```python
from build123d import *

# Parameters (mm, degrees)
SKETCH1_R           = 1.3
SKETCH1_R_2         = 0.3
BOSS_EXTRUDE1_DEPTH = 1
SKETCH1_3_R         = 0.765
BOSS_EXTRUDE2_DEPTH = 0.7
BOSS_EXTRUDE3_DEPTH = 0.6
BOSS_EXTRUDE4_DEPTH = 0.6
BOSS_EXTRUDE5_DEPTH = 0.4
SKETCH5_R           = 0.3
BOSS_EXTRUDE6_DEPTH = 0.4


with BuildPart() as part:
    # Sketch1 → Boss-Extrude1 (new body, symmetric)
    with BuildSketch(Plane.XY):
        Circle(SKETCH1_R)
        Circle(SKETCH1_R_2, mode=Mode.SUBTRACT)
    extrude(amount=BOSS_EXTRUDE1_DEPTH, both=True)



with BuildPart() as body_2:
    # Sketch1_3 → Boss-Extrude2 (new body, symmetric)
    with BuildSketch(Plane.XY):
        with Locations((3.98, -0.68)):
            Circle(SKETCH1_3_R)
    extrude(amount=BOSS_EXTRUDE2_DEPTH, both=True)


with BuildPart() as part_1:
    add(part.part)

    add(body_2.part)  # Boss-Extrude3 merges body 2
    # Sketch1_4 → Boss-Extrude3 (add, symmetric)
    with BuildSketch(Plane.XY):
        with BuildLine():
            ThreePointArc((3.663511304, -1.376462422), (3.215, -0.68), (3.663511304, 0.016462422))
            Line((3.663511304, 0.016462422), (2.68078674, 0.677070497))
            Line((2.68078674, 0.677070497), (0.521604487, 1.190768138))
            ThreePointArc((0.521604487, 1.190768138), (1.088137361, 0.711306603), (1.3, 0))
            ThreePointArc((1.3, 0), (1.133486255, -0.636560217), (0.676601677, -1.110049626))
            add(Edge.make_bspline(
                [(3.663511304, -1.376462422), (2.756337447, -0.967349054), (1.621818, -0.614489974), (0.676601677, -1.110049626)],
                knots=[0, 0, 0, 0, 1, 1, 1, 1], degree=3))
        make_face()
    extrude(amount=BOSS_EXTRUDE3_DEPTH, both=True)

    # Sketch1_5 → Boss-Extrude4 (add, symmetric)
    with BuildSketch(Plane.XY):
        with BuildLine():
            ThreePointArc((-1.295745132, -0.105093068), (-1.071749439, 0.735767042), (-0.36754671, 1.24696007))
            Line((-0.36754671, 1.24696007), (-2.029761859, 2.388087912))
            Line((-2.029761859, 2.388087912), (-3.468005165, 2.793231136))
            Line((-3.468005165, 2.793231136), (-3.852867925, 2.232623737))
            Line((-3.852867925, 2.232623737), (-2.957960282, 1.036034774))
            Line((-2.957960282, 1.036034774), (-1.295745132, -0.105093068))
        make_face()
    extrude(amount=BOSS_EXTRUDE4_DEPTH, both=True)



with BuildPart() as body_2_2:
    # Sketch2 → Revolve1 (revolve)
    with BuildSketch(Plane.XY):
        with BuildLine():
            Line((-3.852867925, 2.232623737), (-3.445366179, 2.826208042))
            Line((-3.445366179, 2.826208042), (-3.775135237, 3.052597901))
            Line((-3.775135237, 3.052597901), (-4.815155649, 1.537660116))
            ThreePointArc((-4.815155649, 1.537660116), (-4.383926247, 1.56515911), (-4.30804714, 1.990549933))
            Line((-4.30804714, 1.990549933), (-3.852867925, 2.232623737))
        make_face()
    revolve(axis=Axis((-3.775135237, 3.052597901, 0), (-0.565974648, -0.824422645, 0)))


with BuildPart() as part_2:
    add(part_1.part)

    add(body_2_2.part)  # Revolve2 merges body 2 2
    # Sketch3 → Revolve2 (revolve)
    with BuildSketch(Plane.XY):
        Polygon((-3.6732598, 3.200993977), (-4.28451242, 2.31061752), (-5.034737027, 2.82565445), (-4.423484407, 3.716030906), align=None)
    revolve(axis=Axis((-3.6732598, 3.200993977, 0), (-0.565974648, -0.824422645, 0)))

    # Sketch4 → Boss-Extrude5 (add)
    with BuildSketch(Plane(origin=(0.316945803, 0.461676681, 0), x_dir=(0.824422645, -0.565974648, 0), z_dir=(0.565974648, 0.824422645, 0))):
        Polygon((-4.84, 0.75055535), (-5.49, 0.375277675), (-5.49, -0.375277675), (-4.84, -0.75055535), (-4.19, -0.375277675), (-4.19, 0.375277675), align=None)
    extrude(amount=BOSS_EXTRUDE5_DEPTH)

    # Sketch5 → Boss-Extrude6 (add)
    with BuildSketch(Plane(origin=(0.543335662, 0.791445739, 0), x_dir=(0.824422645, -0.565974648, 0), z_dir=(0.565974648, 0.824422645, 0))):
        with Locations((-4.84, 0)):
            Circle(SKETCH5_R)
    extrude(amount=BOSS_EXTRUDE6_DEPTH)


solid = part_2.part
```
Geometry: final body of the model. Coordinates: model frame, mm. A direction names the side the tool comes from. Give positions to 0.01 mm unless a question says otherwise; leave off trailing zeros. Loops run counter-clockwise (first coordinate to the right, second up) from the corner with the lowest first, then second, coordinate; pieces in that order, holes last. Notation, with made-up numbers: (24, -14.75) -> (83, -14.75) arc R11 ccw to (83, 2.25) -> close; hole circle Ø3 at (72, -39.5). An arc over 180 degrees is marked (long way). Return JSON: item names as keys, results as strings.
Item 1: Section D-D, the plane y = -0.45. Output: boundary loops of the cut face in (x, z), plus the area to 3 significant figures.
Filled in:
{"outline": "(-1.22, -1) -> (1.22, -1) -> (1.22, -0.6) -> (3.25, -0.6) -> (3.25, -0.7) -> (4.71, -0.7) -> (4.71, 0.7) -> (3.25, 0.7) -> (3.25, 0.6) -> (1.22, 0.6) -> (1.22, 1) -> (-1.22, 1) -> close", "area": "9.36 mm^2"}
Item 2: Access query for faces 1 (the flat face through (4, -1, -0.7)), 2 (the flat face through (4, -1, 0.7)), 3 (the cylindrical face through (-0.28, -1.27, 0.01)). Directions: +Z, -Z, +X, -X, +Y, -Y. A direction counts if a zero-diameter tool reaches every point of the face in a straight line with its end or side. Return the directions, or none.
Filled in:
{"face 1": "-Z, +X, +Y, -Y", "face 2": "+Z, +X, +Y, -Y", "face 3": "none"}
Item 3: Section A-A, the plane x = 0. Output: boundary loops of the cut face in (y, z).
Filled in:
{"outline": "(-1.3, -1) -> (-0.3, -1) -> (-0.3, 1) -> (-1.3, 1) -> close; (0.3, -1) -> (1.3, -1) -> (1.3, 1) -> (0.3, 1) -> close"}
Item 4: Pin query (flat end, axial travel): P1, Ø0.5, axis at x = 4, y = -1, coming from the +Z side; P2, Ø2.5, axis at x = -2.5, y = 2, coming from the +Z side; P3, Ø0.5, axis at x = 4, y = -1, coming from the -Z side. Return the tip coordinate at first contact, or that it passes through.
Filled in:
{"P1": "z = 0.7", "P2": "z = 0.82", "P3": "z = -0.7"}
Item 5: Section B-B, the plane y = 0.9. Output: boundary loops of the cut face in (x, z).
Filled in:
{"outline": "(-2.76, -0.6) -> (-0.94, -0.6) -> (-0.94, -1) -> (0.94, -1) -> (0.94, -0.6) -> (1.74, -0.6) -> (1.74, 0.6) -> (0.94, 0.6) -> (0.94, 1) -> (-0.94, 1) -> (-0.94, 0.6) -> (-2.76, 0.6) -> close"}
Item 6: Section C-C, the plane x = 3.98. Output: boundary loops of the cut face in (y, z) (3 decimals).
Filled in:
{"outline": "(-1.445, -0.7) -> (0.085, -0.7) -> (0.085, 0.7) -> (-1.445, 0.7) -> close"}
Item 7: Line query: line 1 (Y direction, x = 0, z = 0.05); line 2 (Z direction, x = -2.5, y = 2.15); line 3 (X direction, y = 1.6, z = -0.1). Output: solid intervals per line, ascending.
Filled in:
{"line 1": "-1.3 to -0.3, 0.3 to 1.3", "line 2": "-0.6 to 0.6", "line 3": "-4.86 to -4.37, -3.38 to -0.88"}
